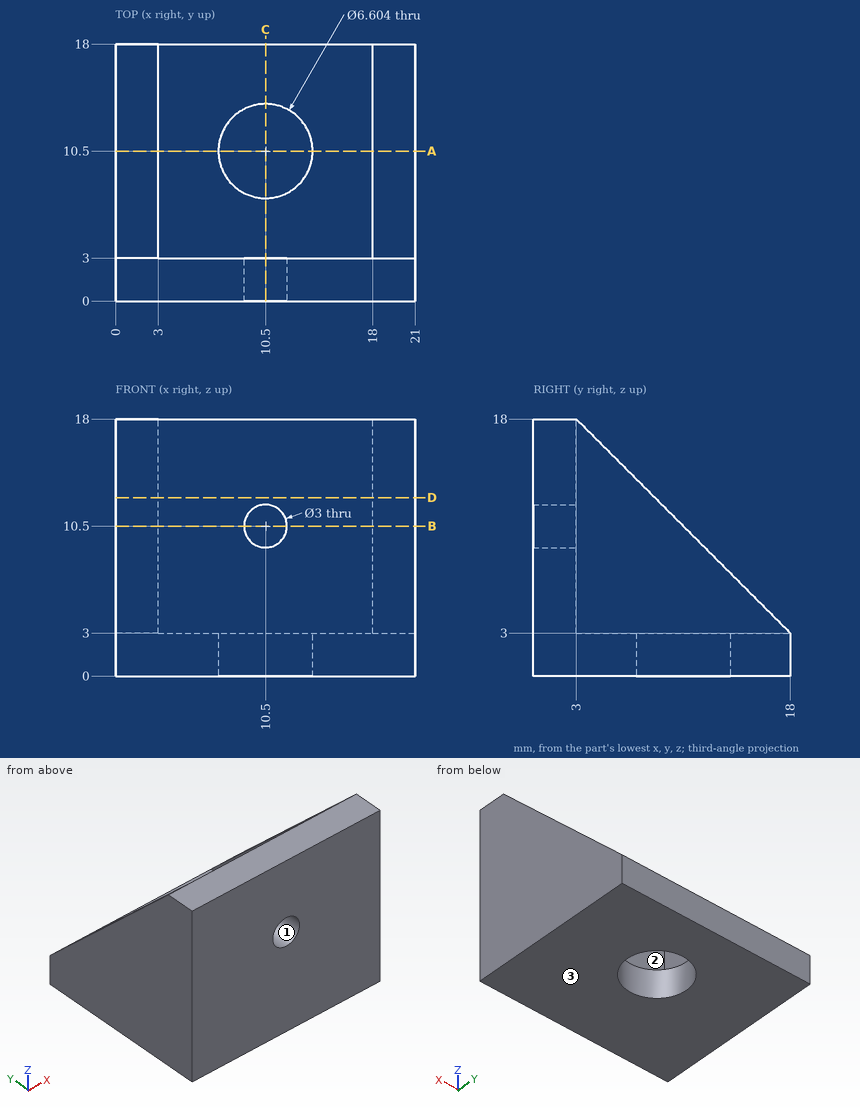
Print and shaded views of the part. All mm, measured from the part's lowest x, y and z. Round coordinates to 2 decimals unless told otherwise and drop trailing zeros. Order: outer loops, then holes, each group sorted by start corner. A loop starts at its lowest first (then second) coordinate and runs counter-clockwise, first axis right, second up.
Q1. Slice it at C-C (x = 10.5). Write the cut outline in (y, z).
Q2. Slice it at B-B (z = 10.5). Write the cut outline in (x, y), and give its area (3 significant figures).
Q3. Wall check: L1, parallel to Y at x = 10.5, z = 2.4; L2, parallel to Z at x = 10.5, y = 2.3; L3, parallel to X at y = 5, z = 5.5. Give the ranges that are in metal, low to high.
Q4. Slice it at D-D (z = 12.5). Write the cut outline in (x, y), and give its area (3 significant figures).
Q5. Drop flat-ended pins along their axis: pin 1 (2 mm diameter, centred on x = 4.5, y = 15, fed in from +Z); pin 2 (3 mm diameter, centred on x = 13, z = 7.5, fed in from +Y). Give the stop position or say it passes through.
Q6. Slice it at A-A (y = 10.5). Write the cut outline in (x, z), and give its area (3 significant figures).
Q7. Two-plate mould, pull along Z, no slides. Class the marked faces 1, 2 and 3: pulls with the +Z half, pulls with the -Z half, needs draft (parallel to the pull), parting line crosses it, or undercut.
Results below:
1. outline: (0, 0) - (7.2, 0) - (7.2, 3) - (3, 3) - (3, 9) - (0, 9) - close; (0, 12) - (3, 12) - (3, 18) - (0, 18) - close; (13.8, 0) - (18, 0) - (18, 3) - (13.8, 3) - close
2. outline: (0, 0) - (9, 0) - (9, 3) - (3, 3) - (3, 10.5) - (0, 10.5) - close; (12, 0) - (21, 0) - (21, 10.5) - (18, 10.5) - (18, 3) - (12, 3) - close
2. area: 99.0 mm2
3. L1: y = 0 to 7.2, 13.8 to 18
3. L2: z = 0 to 9, 12 to 18
3. L3: x = 0 to 3, 18 to 21
4. outline: (0, 0) - (21, 0) - (21, 8.5) - (18, 8.5) - (18, 3) - (3, 3) - (3, 8.5) - (0, 8.5) - close
4. area: 96.0 mm2
5. pin 1: stops at z = 3
5. pin 2: stops at y = 3
6. outline: (0, 0) - (7.2, 0) - (7.2, 3) - (3, 3) - (3, 10.5) - (0, 10.5) - close; (13.8, 0) - (21, 0) - (21, 10.5) - (18, 10.5) - (18, 3) - (13.8, 3) - close
6. area: 88.2 mm2
7. face 1: undercut
7. face 2: needs draft
7. face 3: pulls with the -Z half
